Part model, mm, in its own coordinate system. Face numbers are marked on the shaded views. Give positions to 0.01 mm unless a question says otherwise; leave off trailing zeros. Write each loop counter-clockwise with the first axis right and the second up, starting at its lowest first coordinate (ties: lowest second). Pieces come first, ordered by that corner, then holes. Notation, with made-up numbers: M 17,52 L 48,52 A30 ccw 48,77 Z; hole C -31.5,16 d11. An arc over 180 degrees is marked long. Answer as CSV lines item,"result". Start each with the question number.
1) Slice it at D-D, the plane x = 68. Give the cut face in (y, z), plus the area to 3 significant figures.
2) Slice it at C-C, the plane z = 3. Give the number of separate pieces and of enclosed holes in the cut face, plus the area to 3 significant figures.
3) Wall check: line 1 along X through (y, z) = (-3, -0.5) (1 decimal); line 2 along Z through (x, y) = (0, -16.5); line 3 along X through (y, z) = (-16, -4.5). Give the ranges that are in metal, low to high. Write a range as from..to.
4) Slice it at B-B, the plane y = -27.5. Give the cut face in (x, z), plus the area to 3 significant figures.
5) Slice it at A-A, the plane y = -18.5. Give the cut face in (x, z), plus the area to 3 significant figures.
6) Pin check, flat tips, straight feed: pin 1 Ø12 at (x, z) = (90, 0) entering from -Y; pin 2 Ø4 at (x, y) = (40.5, -25.5) entering from +Z; pin 3 Ø15 at (x, z) = (71.5, 7) entering from -Y; pin 4 Ø1.5 at (y, z) = (-44.5, -5) entering from +X. Stop position of each tip, or through.
7) Mould opens along X. For the marked faces 1, 2 and 3 say: pulls with the +X half, pulls with the -X half, needs draft (parallel to the pull), parting line crosses it, or undercut.
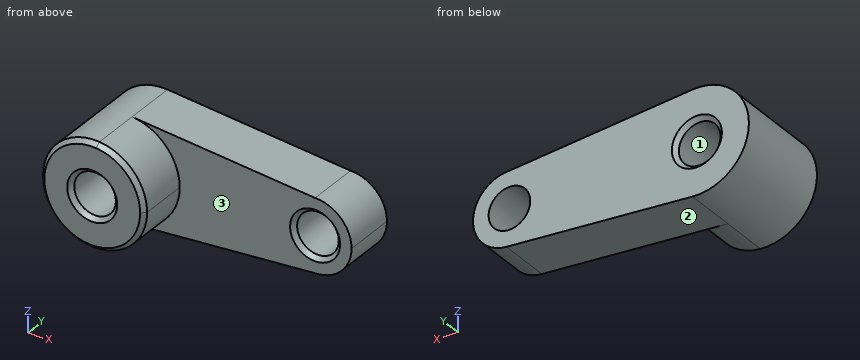
```python
from build123d import *

# Parameters (mm, degrees)
F0_R     = 10
F1_DEPTH = 25
F2_DEPTH = 50
F3_SIZE  = 2


with BuildPart() as f1:
    # F0 (on Front) → F1 (new body)
    with BuildSketch(Plane.XZ):
        with BuildLine():
            ThreePointArc((2.083333, -24.913043), (18.399502, -16.92508), (25, 0))
            ThreePointArc((25, 0), (18.40534, 16.918731), (2.100522, 24.9116))
            ThreePointArc((2.100522, 24.9116), (-24.999999, 0.008625), (2.083333, -24.913043))
        make_face()
        Circle(F0_R, mode=Mode.SUBTRACT)
        with BuildLine():
            ThreePointArc((2.100522, 24.9116), (18.40534, 16.918731), (25, 0))
            ThreePointArc((25, 0), (18.399502, -16.92508), (2.083333, -24.913043))
            Line((2.083333, -24.913043), (91.458333, -17.43913))
            ThreePointArc((91.458333, -17.43913), (72.515224, -0.729802), (90, 17.5))
            Line((90, 17.5), (2.100522, 24.9116))
        make_face()
        with BuildLine():
            ThreePointArc((107.5, 0), (102.374369, 12.374369), (90, 17.5))
            ThreePointArc((90, 17.5), (72.515224, -0.729802), (91.458333, -17.43913))
            ThreePointArc((91.458333, -17.43913), (102.879651, -11.847556), (107.5, 0))
        make_face()
        with Locations((90, 0)):
            Circle(F0_R, mode=Mode.SUBTRACT)
    extrude(amount=F1_DEPTH)

    # F0 (on Front) → F2 (join)
    with BuildSketch(Plane.XZ):
        with BuildLine():
            ThreePointArc((2.083333, -24.913043), (18.399502, -16.92508), (25, 0))
            ThreePointArc((25, 0), (18.40534, 16.918731), (2.100522, 24.9116))
            ThreePointArc((2.100522, 24.9116), (-24.999999, 0.008625), (2.083333, -24.913043))
        make_face()
        Circle(F0_R, mode=Mode.SUBTRACT)
    extrude(amount=F2_DEPTH)

    # F3
    f3_edges = [f1.edges().sort_by_distance(p)[0] for p in [
        (-10, 0, 0),
        (10, -25, 0),
        (-10, -50, 0),
        (-2.083333, -50, 24.913043),
        (80, -25, 0),
    ]]
    chamfer(f3_edges, length=F3_SIZE)


solid = f1.part
```
Found:
1,outline,"M -25,-19.4 L 0,-19.4 L 0,19.36 L -25,19.36 Z"
1,area,"969 mm²"
2,separate pieces,"3"
2,enclosed holes,"0"
2,area,"3,100 mm²"
3,line 1,"-25..-10, 10..80, 100..107.5"
3,line 2,"-25..-10, 10..25"
3,line 3,"-24.59..-8.93, 8.93..81.07, 98.93..106.91"
4,outline,"M 2.08,-24.91 A25 ccw 25,0 A25 ccw long Z; hole C 0,0 d20"
4,area,"1,650 mm²"
5,outline,"M 2.08,-24.91 L 91.46,-17.44 A17.5 ccw 107.5,0 A17.5 ccw 90,17.5 L 2.1,24.91 A25 ccw long Z; hole C 0,0 d20; hole C 90,0 d20"
5,area,"4,670 mm²"
6,pin 1,"through"
6,pin 2,"z = 21.84"
6,pin 3,"y = -25"
6,pin 4,"x = 24.64"
7,face 1,"undercut"
7,face 2,"pulls with the +X half"
7,face 3,"needs draft"
